For this review, take the finished solid that the model builds, in its own axes (mm). Give positions to 0.01 mm unless a question says otherwise; leave off trailing zeros. One line per item, written item: value. Start each with the question number.
from build123d import *

# Parameters (mm, degrees)
EXTRUDE_804_DEPTH        = 0.001
EXTRUDE_804_DEPTH_BACK   = 0.001
SKETCH_6_W               = 5.66
SKETCH_6_H               = 5.96
SWEEP_3_PITCH            = 6.3
SWEEP_3_HEIGHT           = 6.3
SWEEP_3_RADIUS           = 12.25
SWEEP_3_START_ANGLE      = 135
SKETCH_7_W               = 5.7
SKETCH_7_H               = 6
CUT_EXTRUDE_1_DEPTH      = 27.575335967
CUT_EXTRUDE_1_DEPTH_BACK = 27.575335967


with BuildPart() as part:
    # 草图6 → Extrude 804 (new, two sides: drawn at the far end of the back side and taken through both)
    with BuildSketch(Plane(origin=(-8.66205807, 8.66205807, 6.3), x_dir=(0.05768456812732666, 0.057684568127325205, -0.9966669359419564), z_dir=(0.7047499489889816, 0.70474994898897, 0.08157829858529911)).offset(-EXTRUDE_804_DEPTH_BACK)):
        with Locations((2.85, 3)):
            Rectangle(SKETCH_6_W, SKETCH_6_H)
    extrude(amount=EXTRUDE_804_DEPTH + EXTRUDE_804_DEPTH_BACK)

    # 凸台-扫描3: sweep along a helix
    with BuildLine() as sweep_3_path:
        add(Helix(SWEEP_3_PITCH, SWEEP_3_HEIGHT, SWEEP_3_RADIUS, center=(0, 0, 0), direction=(0, 0, 1), lefthand=True, mode=Mode.PRIVATE).rotate(Axis((0, 0, 0), (0, 0, 1)), SWEEP_3_START_ANGLE))
    # 草图7 → 凸台-扫描3 (sweep)
    with BuildSketch(Plane(origin=(-8.66205807, 8.66205807, 6.3), x_dir=(0.05768456812732666, 0.057684568127325205, -0.9966669359419564), z_dir=(0.7047499489889816, 0.70474994898897, 0.08157829858529911))):
        with Locations((2.85, 3)):
            Rectangle(SKETCH_7_W, SKETCH_7_H)
    sweep(path=sweep_3_path.line, is_frenet=True)

    # 草图9 → 切除-拉伸1 (cut, two sides: drawn at the far end of the back side and taken through both)
    with BuildSketch(Plane.XY.offset(-CUT_EXTRUDE_1_DEPTH_BACK)):
        Polygon((-34.190291265, 36.311611608), (0.811494404, 1.30982594), (-1.30982594, -0.811494404), (-38.432931952, 36.311611608), align=None)
    extrude(amount=CUT_EXTRUDE_1_DEPTH + CUT_EXTRUDE_1_DEPTH_BACK, mode=Mode.SUBTRACT)


solid = part.part
Q1. Mouldability with a two-part tool opening along X and no side actions: class faces 1 (the flat face through (-9.7, 11.82, -2.79)), 2 (the flat face through (-11.76, 9.64, 3.3)) as pulls with the +X half, pulls with the -X half, needs draft (parallel to the pull), parting line crosses it, or undercut.
Q2. For line 1 along X through (y, z) = (-4.5, 2.5); line 2 along Y through (x, z) = (-10.5, 3.5); line 3 along X through (y, z) = (5, 1.5), list the stretches that pass through material, from the lowest coordinate up.
Q3. For pin 1 Ø4 at (x, y) = (-13, 3) entering from +Z; pin 2 Ø5 at (x, z) = (-7.5, -2) entering from -Y; pin 3 Ø6 at (x, y) = (13, 6) entering from +Z; pin 4 Ø4 at (y, z) = (14.5, 4.5) entering from +X, all flat-tipped, find the tip position at first contact; note any pin that passes through.
Q4. Take a section at A-A (x = -10.5). State how many separate pieces and enclosed holes the cut face has, and give its area (3 significant figures).
Answers below:
1. face 1: pulls with the -X half
1. face 2: undercut
2. line 1: x = -17.69 to -11.4, 11.39 to 17.69
2. line 2: y = -14.93 to -6.31, 6.31 to 8.38
2. line 3: x = -17.56 to -11.19, 11.18 to 17.55
3. pin 1: stops at z = 5.89
3. pin 2: stops at y = -17.54
3. pin 3: stops at z = 2.14
3. pin 4: passes through
4. separate pieces: 3
4. enclosed holes: 0
4. area: 74.2 mm²
